```python
from build123d import *

# Parameters (mm, degrees)
EXTRUDE_1_DEPTH = 6


with BuildPart() as part:
    # 草图1 → 凸台-拉伸1 (new body)
    with BuildSketch(Plane.XY):
        with BuildLine():
            Line((20, 3), (-20, 3))
            ThreePointArc((-20, 3), (-19.25658351, 1.58113883), (-19, 0))
            ThreePointArc((-19, 0), (-19.25658351, -1.58113883), (-20, -3))
            Line((-20, -3), (20, -3))
            ThreePointArc((20, -3), (19, 0), (20, 3))
        make_face()
        with BuildLine():
            ThreePointArc((-24, -3), (-27, 0), (-24, 3))
            Line((-24, 3), (-20, 3))
            ThreePointArc((-20, 3), (-21.763932022, 4.472135955), (-24, 5))
            ThreePointArc((-24, 5), (-29, 0), (-24, -5))
            ThreePointArc((-24, -5), (-21.763932022, -4.472135955), (-20, -3))
            Line((-20, -3), (-24, -3))
        make_face()
        with BuildLine():
            Line((-20, 3), (-24, 3))
            ThreePointArc((-24, 3), (-21.878679656, 2.121320344), (-21, 0))
            ThreePointArc((-21, 0), (-21.878679656, -2.121320344), (-24, -3))
            Line((-24, -3), (-20, -3))
            ThreePointArc((-20, -3), (-19.25658351, -1.58113883), (-19, 0))
            ThreePointArc((-19, 0), (-19.25658351, 1.58113883), (-20, 3))
        make_face()
        with BuildLine():
            ThreePointArc((24, 5), (21.763932023, 4.472135955), (20, 3))
            Line((20, 3), (24, 3))
            ThreePointArc((24, 3), (26.121320344, 2.121320344), (27, 0))
            ThreePointArc((27, 0), (26.121320344, -2.121320344), (24, -3))
            Line((24, -3), (20, -3))
            ThreePointArc((20, -3), (21.763931997, -4.472135942), (23.999999943, -5))
            ThreePointArc((23.999999943, -5), (27.535533886, -3.535533926), (29, 0))
            ThreePointArc((29, 0), (27.535533906, 3.535533906), (24, 5))
        make_face()
        with BuildLine():
            Line((24, 3), (20, 3))
            ThreePointArc((20, 3), (19, 0), (20, -3))
            Line((20, -3), (24, -3))
            ThreePointArc((24, -3), (21, 0), (24, 3))
        make_face()
    extrude(amount=EXTRUDE_1_DEPTH)


solid = part.part
```
Geometry: final body of the model. Coordinates: model frame, mm. A direction names the side the tool comes from. Give positions to 0.01 mm unless a question says otherwise; leave off trailing zeros. Loops run counter-clockwise (first coordinate to the right, second up) from the corner with the lowest first, then second, coordinate; pieces in that order, holes last. Notation, with made-up numbers: (4.5, 41.5) -> (11.5, 41.5) arc R26 cw to (11.5, 79.5) -> close; hole circle Ø6 at (-23, -14). An arc over 180 degrees is marked (long way). Return JSON: item names as keys, results as strings.
Item 1: Section C-C, the plane x = 0.5. Output: boundary loops of the cut face in (y, z), plus the area to 3 significant figures.
Filled in:
{"outline": "(-3, 0) -> (3, 0) -> (3, 6) -> (-3, 6) -> close", "area": "36.0 mm^2"}
Item 2: Access query for faces 3 (the flat face through (0, 0, 0)), 4 (the flat face through (0, 3, 3)). Directions: +Z, -Z, +X, -X, +Y, -Y. A direction counts if a zero-diameter tool reaches every point of the face in a straight line with its end or side. Return the directions, or none.
Filled in:
{"face 3": "-Z, +X, -X, +Y, -Y", "face 4": "+Z, -Z, +Y"}
Item 3: Line query: line 1 (X direction, y = -2.75, z = 5.55); line 2 (X direction, y = 1, z = 2.7); line 3 (Y direction, x = 25, z = 2.4). Output: solid intervals per line, ascending.
Filled in:
{"line 1": "-28.18 to -25.2, -22.8 to 22.8, 25.2 to 28.18", "line 2": "-28.9 to -26.83, -21.17 to 21.17, 26.83 to 28.9", "line 3": "-4.9 to -2.83, 2.83 to 4.9"}
Item 4: Section B-B, the plane y = 4.25. Output: boundary loops of the cut face in (x, z).
Filled in:
{"outline": "(-26.63, 0) -> (-21.37, 0) -> (-21.37, 6) -> (-26.63, 6) -> close; (21.37, 0) -> (26.63, 0) -> (26.63, 6) -> (21.37, 6) -> close"}
Item 5: Pin query (flat end, axial travel): P1, Ø3, axis at x = 7, z = 2, coming from the +Y side. Return the tip coordinate at first contact, or that it passes through.
Filled in:
{"P1": "y = 3"}
Item 6: Section A-A, the plane z = 3.35. Output: boundary loops of the cut face in (x, y).
Filled in:
{"outline": "(-20, -3) -> (20, -3) arc R5 ccw (long way) to (20, 3) -> (-20, 3) arc R5 ccw (long way) to start; hole circle Ø6 at (-24, 0); hole circle Ø6 at (24, 0)"}
Item 7: Mould query, pull axis X, two halves, no side actions, for faces 1 (the flat face through (0, -3, 3)), 2 (the flat face through (0, 0, 6)). Classes: released by +X, released by -X, zero draft, split by the parting line, or undercut.
Filled in:
{"face 1": "undercut", "face 2": "zero draft"}
